Could you check a few things on this drawing? It's one solid part, dimensions in mm from its lowest x, y, z. Give positions to 0.01 mm unless a question says otherwise; leave off trailing zeros. Order: outer loops, then holes, each group sorted by start corner. A loop starts at its lowest first (then second) coordinate and runs counter-clockwise, first axis right, second up. Notation, with made-up numbers: (-30.5, 73) - (-11.5, 73) arc R12 ccw to (-11.5, 96) - close; hole circle Ø5 at (87.25, -12.75). An arc over 180 degrees is marked (long way). Return JSON: item names as keys, results as strings.
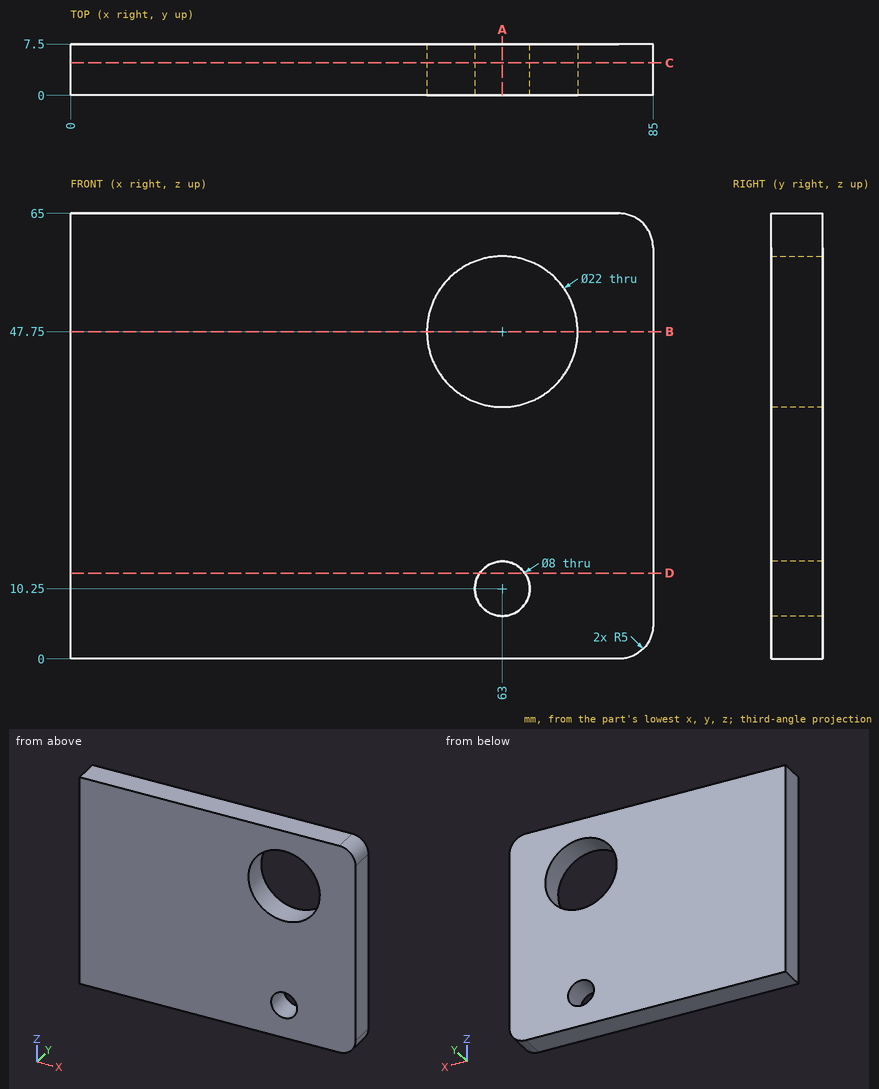
1. Suppose I cut it at C-C (y = 4.75). List the corners of the cut face in (x, z) for me.
Checks:
{"outline": "(0, 0) - (80, 0) arc R5 ccw to (85, 5) - (85, 60) arc R5 ccw to (80, 65) - (0, 65) - close; hole circle Ø22 at (63, 47.75); hole circle Ø8 at (63, 10.25)"}
2. For pin 1 Ø6.5 at (x, z) = (63, 10.25) entering from +Y, with a flat end and sliding along its axis, tell me the tip position at first contact or that it passes through.
Checks:
{"pin 1": "through"}
3. If I drill on L1, parallel to Z at x = 63, y = 5.75; L2, parallel to X at y = 3.75, z = 47.75; L3, parallel to X at y = 2.5, z = 10.25, over which ranges is the centre line in solid material (lowest first)? Write a range as [from, to].
Checks:
{"L1": "[0, 6.25], [14.25, 36.75], [58.75, 65]", "L2": "[0, 52], [74, 85]", "L3": "[0, 59], [67, 85]"}
4. Suppose I cut it at A-A (x = 63). List the corners of the cut face in (y, z) for me.
Checks:
{"outline": "(0, 0) - (7.5, 0) - (7.5, 6.25) - (0, 6.25) - close; (0, 14.25) - (7.5, 14.25) - (7.5, 36.75) - (0, 36.75) - close; (0, 58.75) - (7.5, 58.75) - (7.5, 65) - (0, 65) - close"}
5. Suppose I cut it at D-D (z = 12.5). List the corners of the cut face in (x, y) for me, plus the area to 3 significant figures.
Checks:
{"outline": "(0, 0) - (59.69, 0) - (59.69, 7.5) - (0, 7.5) - close; (66.31, 0) - (85, 0) - (85, 7.5) - (66.31, 7.5) - close", "area": "588 mm^2"}
6. Suppose I cut it at B-B (z = 47.75). List the corners of the cut face in (x, y) for me.
Checks:
{"outline": "(0, 0) - (52, 0) - (52, 7.5) - (0, 7.5) - close; (74, 0) - (85, 0) - (85, 7.5) - (74, 7.5) - close"}
